Input: dimensioned drawing with shaded views. Units: mm. Origin: part minimum x, y, z. A direction names the side the tool comes from. Give positions to 0.01 mm unless a question says otherwise; leave off trailing zeros. Order: outer loops, then holes, each group sorted by start corner. A loop starts at its lowest first (then second) coordinate and runs counter-clockwise, first axis right, second up. Notation, with made-up numbers: M -40,-18.5 L -7,-18.5 A14 ccw -7,-12.5 Z; hole C -29.75,0.5 d4. An arc over 180 degrees is marked long. Answer in a Markdown table with one row per item. Add a question column.
(1) Material intervals for line 1 along Y through (x, z) = (5, 6); line 2 along Z through (x, y) = (4.5, 8.25); line 3 along Y through (x, z) = (3.5, 1.25), sorted ascending.
(2) Mould query, pull axis Y, two halves, no side actions, for the marked faces 3, 4 and 5. Classes: pulls with the +Y half, pulls with the -Y half, needs draft (parallel to the pull), parting line crosses it, or undercut.
(3) Pin query (flat end, axial travel): P1, Ø3, axis at x = 5, y = 3.5, coming from the +Z side; P2, Ø1.5, axis at x = 6.5, z = 6, coming from the +Y side; P3, Ø5, axis at x = 1, z = 5.5, coming from the -Y side; P4, Ø3, axis at x = 9, z = 1, coming from the -Y side. Return the tip coordinate at first contact, or that it passes through.
(4) Section query C-C, the plane z = 8.75. Return loops of the section in (x, y), plus the area to 3 significant figures.
(5) Section query A-A, the plane y = 5. Return loops of the section in (x, z).
(6) Set-up query: the marked faces 1 and 2. Return all of +Z, -Z, +X, -X, +Y, -Y with unobstructed straight access to the full face (end or side cutting, diameter ignored); none if empty.
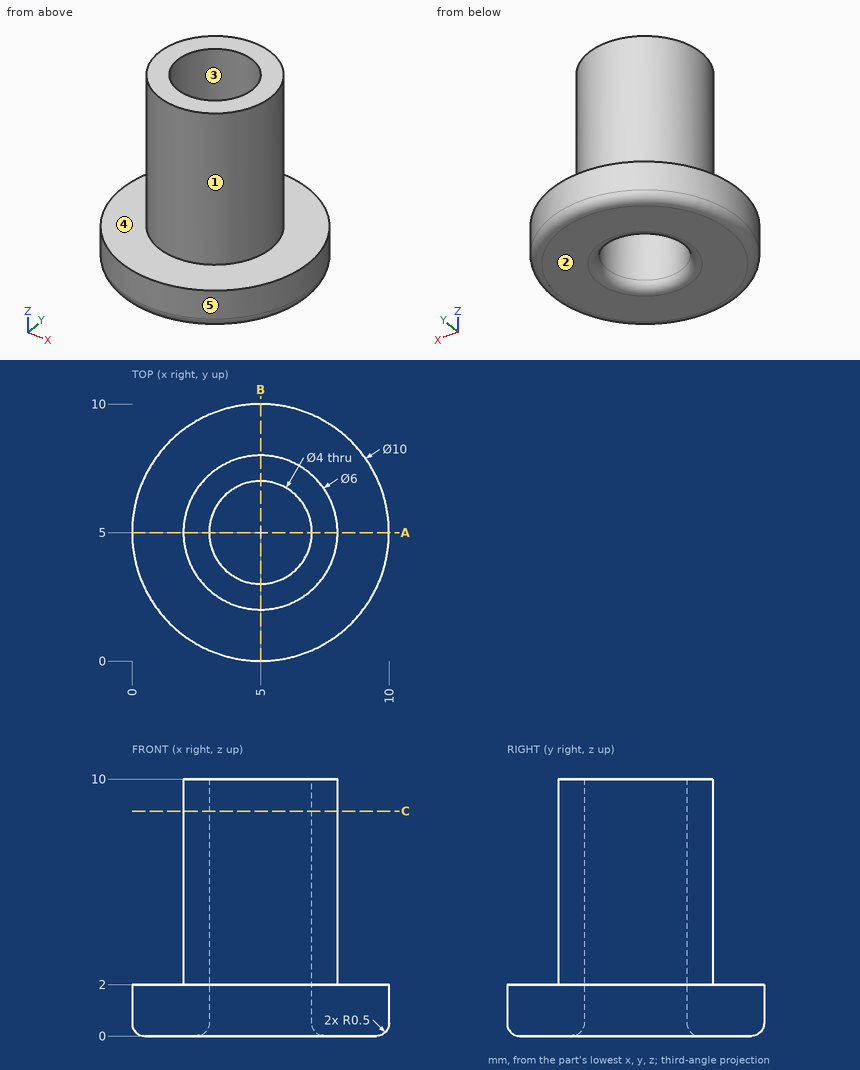
Values follow:
| question | item | result |
|---|---|---|
| 1 | line 1 | y = 2 to 3, 7 to 8 |
| 1 | line 2 | z = 0 to 2 |
| 1 | line 3 | y = 0.23 to 3.68, 6.32 to 9.77 |
| 2 | face 3 | undercut |
| 2 | face 4 | needs draft |
| 2 | face 5 | parting line crosses it |
| 3 | P1 | stops at z = 10 |
| 3 | P2 | stops at y = 7.9 |
| 3 | P3 | stops at y = 2.4 |
| 3 | P4 | stops at y = 0.67 |
| 4 | outline | C 5,5 d6; hole C 5,5 d4 |
| 4 | area | 15.7 mm² |
| 5 | outline | M 0,0.5 A0.5 ccw 0.5,0 L 2.5,0 A0.5 ccw 3,0.5 L 3,10 L 2,10 L 2,2 L 0,2 Z; M 7,0.5 A0.5 ccw 7.5,0 L 9.5,0 A0.5 ccw 10,0.5 L 10,2 L 8,2 L 8,10 L 7,10 Z |
| 6 | face 1 | +Z |
| 6 | face 2 | -Z, +X, -X, +Y, -Y |
